Drawing for the job (mm, zero at the part's lowest x, y, z). A direction names the side the tool comes from. Round coordinates to 2 decimals unless told otherwise and drop trailing zeros. Write each loop counter-clockwise with the first axis right and the second up, starting at its lowest first coordinate (ties: lowest second). Pieces come first, ordered by that corner, then holes.
Item 1: Band-saw the part on A-A, the plane y = 11.25. Write the cut outline in (x, z) (3 decimals), then the cut area to 3 significant figures.
Item 2: Band-saw the part on D-D, the plane x = 120.5. Write the cut outline in (y, z) (3 decimals), then the cut area to 3 significant figures.
Item 3: 3-axis set-ups, long thin cutter, end or side, ignore diameter. For the marked faces 1, 2 and 3: which of +Z, -Z, +X, -X, +Y, -Y reach the whole face in a straight line?
Item 4: Band-saw the part on C-C, the plane x = 16.51. Write the cut outline in (y, z), then the cut area to 3 significant figures.
Item 5: Mould opens along X. For the marked faces 4 and 5 say: +X half, -X half, draft (parallel to the pull), parting line (faces both ways), or undercut.
Item 6: Wall check: probe 1 along X at (y, z) = (8, 16.5); probe 2 along X at (y, z) = (4, 21.5); probe 3 along Z at (x, y) = (92, 6.5) (3 decimals). Give the ranges that are in metal, low to high.
Item 7: Band-saw the part on B-B, the plane z = 21. Write the cut outline in (x, y).
Item 8: Drop flat-ended pins along their axis: pin 1 Ø6 at (x, z) = (122.5, 12) entering from -Y; pin 2 Ø5 at (y, z) = (6.5, 10) entering from -X; pin 3 Ø2 at (y, z) = (6.5, 4.5) entering from -X; pin 4 Ø3 at (x, y) = (123.5, 9) entering from +Z (3 decimals). Give the stop position or say it passes through.
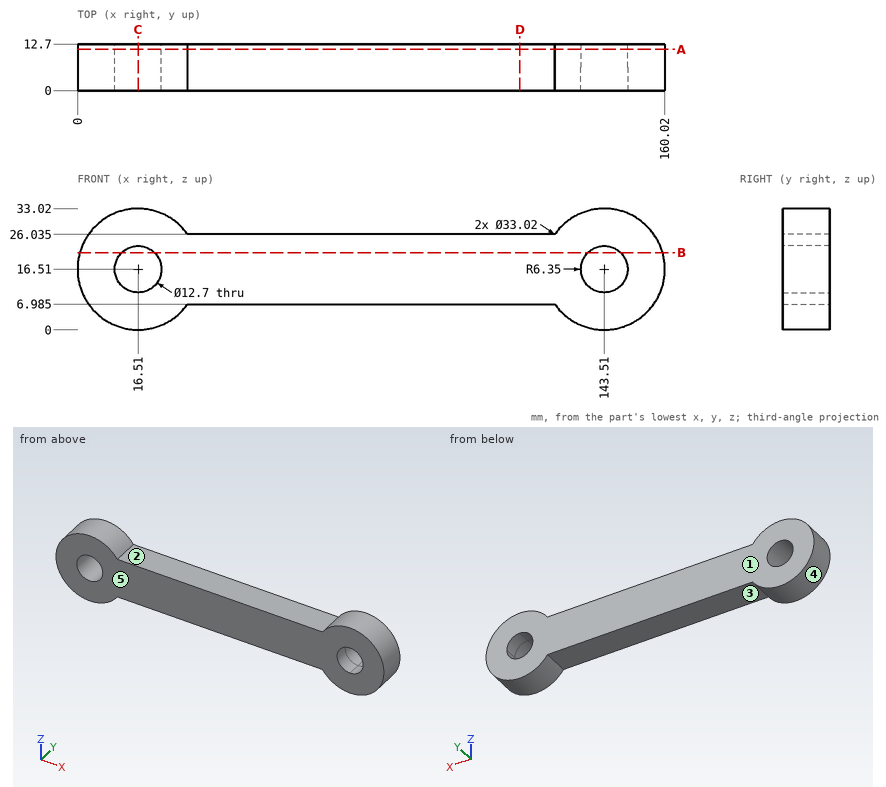
Results:
1. outline: (29.995, 6.985) - (130.025, 6.985) arc R16.51 ccw (long way) to (130.025, 26.035) - (29.995, 26.035) arc R16.51 ccw (long way) to start; hole circle Ø12.7 at (16.51, 16.51); hole circle Ø12.7 at (143.51, 16.51)
1. area: 3,290 mm2
2. outline: (0, 6.985) - (12.7, 6.985) - (12.7, 26.035) - (0, 26.035) - close
2. area: 242 mm2
3. face 1: +Z, -Z, +X, -X, +Y
3. face 2: +Z, +Y, -Y
3. face 3: -Z, +Y, -Y
4. outline: (0, 0) - (12.7, 0) - (12.7, 10.16) - (0, 10.16) - close; (0, 22.86) - (12.7, 22.86) - (12.7, 33.02) - (0, 33.02) - close
4. area: 258 mm2
5. face 4: undercut
5. face 5: draft
6. probe 1: x = 0 to 10.16, 22.86 to 137.16, 149.86 to 160.02
6. probe 2: x = 0.77 to 12.58, 20.44 to 139.58, 147.44 to 159.25
6. probe 3: z = 6.985 to 26.035
7. outline: (0.62, 0) - (12.02, 0) - (12.02, 12.7) - (0.62, 12.7) - close; (21, 0) - (139.02, 0) - (139.02, 12.7) - (21, 12.7) - close; (148, 0) - (159.4, 0) - (159.4, 12.7) - (148, 12.7) - close
8. pin 1: stops at y = 0
8. pin 2: stops at x = 0.49
8. pin 3: stops at x = 4.21
8. pin 4: stops at z = 26.035
